Build history of the part. All positions in model axes, mm. Round coordinates to 2 decimals unless told otherwise and drop trailing zeros. Order: outer loops, then holes, each group sorted by start corner. A loop starts at its lowest first (then second) coordinate and runs counter-clockwise, first axis right, second up. Notation, with made-up numbers: M -10,70 L 11,70 A5 ccw 11,76 Z; hole C -32,50 d3. An arc over 180 degrees is marked long. One line per question, with ' | ' between items. Start each with the question number.
from build123d import *
from build123d.topology import SkipClean

# Parameters (mm, degrees)
SKETCH1_R           = 6.5
BOSS_EXTRUDE1_DEPTH = 4
SKETCH2_R           = 6.5
BOSS_EXTRUDE2_DEPTH = 8
SKETCH3_R           = 4.25
CUT_EXTRUDE4_DEPTH  = 48.299577165
CHAMFER2_SIZE       = 0.2
CHAMFER3_SIZE       = 0.5


with BuildPart() as part:
    # Sketch1 → Boss-Extrude1 (new, symmetric)
    with BuildSketch(Plane.XY):
        with BuildLine():
            Line((-6.5, -21), (-6.5, 21))
            ThreePointArc((-6.5, 21), (-3.057753594, 26.735864622), (3.62312091, 26.396572512))
            Line((3.62312091, 26.396572512), (30.574032169, 8.302419249))
            ThreePointArc((30.574032169, 8.302419249), (35, 0), (30.574032169, -8.302419249))
            Line((30.574032169, -8.302419249), (3.62312091, -26.396572512))
            ThreePointArc((3.62312091, -26.396572512), (-3.057753594, -26.735864622), (-6.5, -21))
        make_face()
        with Locations((25, 0)):
            Circle(SKETCH1_R, mode=Mode.SUBTRACT)
    extrude(amount=BOSS_EXTRUDE1_DEPTH, both=True)

    # Sketch2 → Boss-Extrude2 (add, symmetric)
    with SkipClean():  # the faces are left unmerged after this step: merging them gives an invalid solid
        with BuildSketch(Plane.XY):
            with Locations((0, 21)):
                Circle(SKETCH2_R)
            with Locations((0, -21)):
                Circle(SKETCH2_R)
        extrude(amount=BOSS_EXTRUDE2_DEPTH, both=True)
    add(part.part.scale(1), mode=Mode.REPLACE)  # the faces are merged on a copy

    # Sketch3 → Cut-Extrude4 (cut, through all)
    with BuildSketch(Plane.XY.offset(8)):
        with Locations((0, 21)):
            Circle(SKETCH3_R)
        with Locations((0, -21)):
            Circle(SKETCH3_R)
    extrude(amount=-CUT_EXTRUDE4_DEPTH, mode=Mode.SUBTRACT)

    # Chamfer2
    chamfer2_edges = [part.edges().sort_by_distance(p)[0] for p in [
        (-6.5, 21, -8),
        (-6.5, 21, 8),
        (-6.5, -21, -8),
        (-6.5, -21, 8),
        (-4.25, 21, -8),
        (-4.25, 21, 8),
        (-4.25, -21, -8),
        (-4.25, -21, 8),
    ]]
    chamfer(chamfer2_edges, length=CHAMFER2_SIZE)

    # Chamfer3
    # the kernel refuses this chamfer: 0.5 mm, written as the material it takes off along each edge
    with BuildSketch(Plane(origin=(25, 0, 4), x_dir=(0.557403216886901, 0.8302419248653579, 0), z_dir=(-0.8302419248653579, 0.557403216886901, 0))) as chamfer3_piece_1:
        Polygon((10, CHAMFER3_SIZE), (10 - CHAMFER3_SIZE, 0), (10, 0), align=None)
    revolve(axis=Axis((25, 0, 4), (0, 0, -1)), revolution_arc=112.247195119, mode=Mode.SUBTRACT)
    with BuildSketch(Plane(origin=(2.555561393, 27.113304697, 4), x_dir=(0.01532629007386634, 0.022828229523033896, -0.9996219169112968), z_dir=(0.8302419248653579, -0.5574032168869009, 0))) as chamfer3_piece_2_section:
        Polygon((CHAMFER3_SIZE * 0.999621916911, -CHAMFER3_SIZE * 0.0274958766106), (-CHAMFER3_SIZE * 0.0274958766106, -CHAMFER3_SIZE * 0.999621916911), (0, 0), align=None)
    chamfer3_piece_2 = extrude(amount=33.74735717, mode=Mode.PRIVATE)
    chamfer3_piece_2 = chamfer3_piece_2 - Plane(origin=(0, 21, 3.833161129), x_dir=(1, 0, 0), z_dir=(0, 0, 1)) * Cylinder(6.5, 70, mode=Mode.PRIVATE)
    add(chamfer3_piece_2, mode=Mode.SUBTRACT)
    with BuildSketch(Plane(origin=(25, 0, -4), x_dir=(1, 0, 0), z_dir=(0, -1, 0))) as chamfer3_piece_3:
        Polygon((6.5 + CHAMFER3_SIZE, 0), (6.5, CHAMFER3_SIZE), (6.5, 0), align=None)
    revolve(axis=Axis((25, 0, -4), (0, 0, 1)), mode=Mode.SUBTRACT)
    with BuildSketch(Plane(origin=(25, 0, 4), x_dir=(1, 0, 0), z_dir=(0, -1, 0))) as chamfer3_piece_4:
        Polygon((6.5, -CHAMFER3_SIZE), (6.5 + CHAMFER3_SIZE, 0), (6.5, 0), align=None)
    revolve(axis=Axis((25, 0, 4), (0, 0, 1)), mode=Mode.SUBTRACT)
    with BuildSketch(Plane(origin=(-6.5, -22.285841494, 4), x_dir=(-0.027495876610585623, 0, -0.9996219169112968), z_dir=(0, 1, 0))) as chamfer3_piece_5_section:
        Polygon((CHAMFER3_SIZE * 0.999621916911, -CHAMFER3_SIZE * 0.0274958766106), (-CHAMFER3_SIZE * 0.0274958766106, -CHAMFER3_SIZE * 0.999621916911), (0, 0), align=None)
    chamfer3_piece_5 = extrude(amount=44.571682988, mode=Mode.PRIVATE)
    chamfer3_piece_5 = chamfer3_piece_5 - Plane(origin=(0, -21, 3.832044631), x_dir=(1, 0, 0), z_dir=(0, 0, 1)) * Cylinder(6.5, 92, mode=Mode.PRIVATE)
    chamfer3_piece_5 = chamfer3_piece_5 - Plane(origin=(0, 21, 3.832044631), x_dir=(1, 0, 0), z_dir=(0, 0, 1)) * Cylinder(6.5, 92, mode=Mode.PRIVATE)
    add(chamfer3_piece_5, mode=Mode.SUBTRACT)
    with BuildSketch(Plane(origin=(-6.5, -22.285841494, -4), x_dir=(0.9996219169112968, 0, -0.027495876610585647), z_dir=(0, 1, 0))) as chamfer3_piece_6_section:
        Polygon((CHAMFER3_SIZE * 0.999621916911, -CHAMFER3_SIZE * 0.0274958766106), (-CHAMFER3_SIZE * 0.0274958766106, -CHAMFER3_SIZE * 0.999621916911), (0, 0), align=None)
    chamfer3_piece_6 = extrude(amount=44.571682988, mode=Mode.PRIVATE)
    chamfer3_piece_6 = chamfer3_piece_6 - Plane(origin=(0, -21, -3.832044585), x_dir=(1, 0, 0), z_dir=(0, 0, 1)) * Cylinder(6.5, 92, mode=Mode.PRIVATE)
    chamfer3_piece_6 = chamfer3_piece_6 - Plane(origin=(0, 21, -3.832044585), x_dir=(1, 0, 0), z_dir=(0, 0, 1)) * Cylinder(6.5, 92, mode=Mode.PRIVATE)
    add(chamfer3_piece_6, mode=Mode.SUBTRACT)
    with BuildSketch(Plane(origin=(2.555561393, 27.113304697, -4), x_dir=(-0.5571924721570072, -0.8299280244340339, -0.027495876610585664), z_dir=(0.8302419248653579, -0.5574032168869009, 0))) as chamfer3_piece_7_section:
        Polygon((CHAMFER3_SIZE * 0.999621916911, -CHAMFER3_SIZE * 0.0274958766106), (-CHAMFER3_SIZE * 0.0274958766106, -CHAMFER3_SIZE * 0.999621916911), (0, 0), align=None)
    chamfer3_piece_7 = extrude(amount=33.74735717, mode=Mode.PRIVATE)
    chamfer3_piece_7 = chamfer3_piece_7 - Plane(origin=(0, 21, -3.833161129), x_dir=(1, 0, 0), z_dir=(0, 0, 1)) * Cylinder(6.5, 70, mode=Mode.PRIVATE)
    add(chamfer3_piece_7, mode=Mode.SUBTRACT)
    with BuildSketch(Plane(origin=(25, 0, -4), x_dir=(0.557403216886901, 0.8302419248653579, 0), z_dir=(-0.8302419248653579, 0.557403216886901, 0))) as chamfer3_piece_8:
        Polygon((10 - CHAMFER3_SIZE, 0), (10, -CHAMFER3_SIZE), (10, 0), align=None)
    revolve(axis=Axis((25, 0, -4), (0, 0, -1)), revolution_arc=112.247195119, mode=Mode.SUBTRACT)
    with BuildSketch(Plane(origin=(30.574032169, -8.302419249, -4), x_dir=(-0.5571924721570071, 0.8299280244340339, -0.027495876610585612), z_dir=(-0.8302419248653579, -0.5574032168869009, 0))) as chamfer3_piece_9_section:
        Polygon((CHAMFER3_SIZE * 0.999621916911, -CHAMFER3_SIZE * 0.0274958766106), (-CHAMFER3_SIZE * 0.0274958766106, -CHAMFER3_SIZE * 0.999621916911), (0, 0), align=None)
    chamfer3_piece_9 = extrude(amount=33.74735717, mode=Mode.PRIVATE)
    chamfer3_piece_9 = chamfer3_piece_9 - Plane(origin=(0, -21, -3.833161128), x_dir=(1, 0, 0), z_dir=(0, 0, 1)) * Cylinder(6.5, 70, mode=Mode.PRIVATE)
    add(chamfer3_piece_9, mode=Mode.SUBTRACT)
    with BuildSketch(Plane(origin=(30.574032169, -8.302419249, 4), x_dir=(0.015326290073865267, -0.022828229523032303, -0.9996219169112968), z_dir=(-0.8302419248653579, -0.5574032168869009, 0))) as chamfer3_piece_10_section:
        Polygon((CHAMFER3_SIZE * 0.999621916911, -CHAMFER3_SIZE * 0.0274958766106), (-CHAMFER3_SIZE * 0.0274958766106, -CHAMFER3_SIZE * 0.999621916911), (0, 0), align=None)
    chamfer3_piece_10 = extrude(amount=33.74735717, mode=Mode.PRIVATE)
    chamfer3_piece_10 = chamfer3_piece_10 - Plane(origin=(0, -21, 3.833161129), x_dir=(1, 0, 0), z_dir=(0, 0, 1)) * Cylinder(6.5, 70, mode=Mode.PRIVATE)
    add(chamfer3_piece_10, mode=Mode.SUBTRACT)


solid = part.part
Item 1: Wall check: line 1 along Y through (x, z) = (0, -0.5); line 2 along Z through (x, y) = (-0.5, 0); line 3 along Y through (x, z) = (-3.5, -2). Give the ranges that are in metal, low to high. Write a range as [from, to].
Item 2: Cut at C-C on z = -2.5. Write the cut outline in (x, y), then the cut area to 3 significant figures.
Item 3: Cut at A-A on z = 6. Write the cut outline in (x, y).
Item 4: Cut at D-D on x = 0. Count the separate pieces of the cut face and the enclosed holes in it, then the cut area to 3 significant figures.
Item 5: Two-plate mould, pull along X, no slides. Class faces 1 (the face through (18.506, 0.286, -0.049)), 2 (the face through (10, 0, 4)), 3 (the face through (17.29, -17.22, 0.05)): +X half, -X half, draft (parallel to the pull), parting line (faces both ways), or undercut.
Item 6: Flat gauge pins, fed straight in: pin 1 (12 mm diameter, centred on x = 6.5, y = 8.5, fed in from +Z); pin 2 (3 mm diameter, centred on x = 14, y = 17.5, fed in from -Z); pin 3 (7.5 mm diameter, centred on x = 0, y = 21, fed in from -Z); pin 4 (6 mm diameter, centred on y = -7, z = -2.5, fed in from +X). Where does each tip first touch, or does it go through?
Item 7: Cut at B-B on x = 25. Write the cut outline in (y, z).
Results found:
1) line 1: y = [-27.5, -25.25], [-16.75, 16.75], [25.25, 27.5] | line 2: z = [-4, 4] | line 3: y = [-26.48, -23.41], [-18.59, 18.59], [23.41, 26.48]
2) outline: M -6.5,-21 A6.5 ccw 3.62,-26.4 L 30.57,-8.3 A10 ccw 30.57,8.3 L 3.62,26.4 A6.5 ccw -6.5,21 Z; hole C 0,-21 d8.5; hole C 0,21 d8.5; hole C 25,0 d13 | area: 1,280 mm^2
3) outline: C 0,-21 d13; C 0,21 d13; hole C 0,-21 d8.5; hole C 0,21 d8.5
4) separate pieces: 3 | enclosed holes: 0 | area: 376 mm^2
5) face 1: undercut | face 2: draft | face 3: +X half
6) pin 1: stops at z = 4 | pin 2: stops at z = -4 | pin 3: passes through | pin 4: stops at x = 34.17
7) outline: M -12.04,-3.5 L -11.44,-4 L -7,-4 L -6.5,-3.5 L -6.5,3.5 L -7,4 L -11.44,4 L -12.04,3.5 Z; M 6.5,-3.5 L 7,-4 L 11.44,-4 L 12.04,-3.5 L 12.04,3.5 L 11.44,4 L 7,4 L 6.5,3.5 Z
